Part model, mm, in its own coordinate system. A direction names the side the tool comes from. Round coordinates to 2 decimals unless told otherwise and drop trailing zeros. Order: outer loops, then holes, each group sorted by start corner. A loop starts at its lowest first (then second) coordinate and runs counter-clockwise, first axis right, second up. Notation, with made-up numbers: M 85.25,74 L 103.25,74 A15 ccw 103.25,100 Z; hole C -31,55.5 d2. An arc over 180 degrees is marked long. Write each question's results on one line, items separated by ' | '. Start each with the question number.
1. Band-saw the part on B-B, the plane z = -64. List the corners of the cut face in (x, y), then the cut area to 3 significant figures.
2. Probe L1, parallel to X at y = 5.75, z = -88; L2, parallel to X at y = 3.25, z = -13; L3, parallel to Z at x = 39, y = 8.25. List the from-to ranges inside material, lowest first. Write a range as [from, to].
3. Which spindle directions (+Z, -Z, +X, -X, +Y, -Y) get a long thin tool onto all of the face, cutting with end or side? Do faces 1 (the face through (6, 7, -49)), 2 (the face through (82, 7, -6)), 3 (the face through (70, 5, -88)), 4 (the face through (30, 5, -12)), 5 (the face through (18, 7, -94)). Say none if no direction does.
4. Two-plate mould, pull along X, no slides. Class faces 6 (the face through (100, 2, -49)), 7 (the face through (15, 2, 0)), 8 (the face through (50, 5, -20)): +X half, -X half, draft (parallel to the pull), parting line (faces both ways), or undercut.
5. Band-saw the part on C-C, the plane x = 11.5. List the corners of the cut face in (y, z).
6. Band-saw the part on D-D, the plane y = 3. List the corners of the cut face in (x, z).
7. Drop flat-ended pins along their axis: pin 1 Ø1.5 at (x, y) = (49, 6.5) entering from +Z; pin 2 Ø4 at (x, y) = (88, 8.5) entering from -Z; pin 3 Ø4 at (y, z) = (8.5, -66) entering from -X. Give the stop position or say it passes through.
8. Band-saw the part on A-A, the plane z = -13. List the corners of the cut face in (x, y).
```python
from build123d import *

# Parameters (mm, degrees)
SKETCH1_W           = 100
SKETCH1_H           = 100
BOSS_EXTRUDE1_DEPTH = 5
SKETCH2_W           = 88
SKETCH2_H           = 88
BOSS_EXTRUDE2_DEPTH = 5
SKETCH3_W           = 40
SKETCH3_H           = 20
CUT_EXTRUDE1_DEPTH  = 10


with BuildPart() as part:
    # Sketch1 → Boss-Extrude1 (new body)
    with BuildSketch(Plane(origin=(0, 0, 0), x_dir=(1, 0, 0), z_dir=(0, 1, 0))):
        with Locations((50, 50)):
            Rectangle(SKETCH1_W, SKETCH1_H)
    extrude(amount=BOSS_EXTRUDE1_DEPTH)

    # Sketch2 → Boss-Extrude2 (add)
    with BuildSketch(Plane(origin=(0, 5, 0), x_dir=(1, 0, 0), z_dir=(0, 1, 0))):
        with Locations((50, 50)):
            Rectangle(SKETCH2_W, SKETCH2_H)
    extrude(amount=BOSS_EXTRUDE2_DEPTH)

    # Sketch3 → Cut-Extrude1 (cut)
    with BuildSketch(Plane.XZ):
        with Locations((50, -90)):
            Rectangle(SKETCH3_W, SKETCH3_H)
        with Locations((50, -10)):
            Rectangle(SKETCH3_W, SKETCH3_H)
    extrude(amount=-CUT_EXTRUDE1_DEPTH, mode=Mode.SUBTRACT)


solid = part.part
```
Solution:
1) outline: M 0,0 L 100,0 L 100,5 L 94,5 L 94,10 L 6,10 L 6,5 L 0,5 Z | area: 940 mm^2
2) L1: [6, 30], [70, 94] | L2: [0, 30], [70, 100] | L3: [-80, -20]
3) face 1: +Z, -Z, -X, +Y | face 2: +Z, +X, -X, +Y | face 3: -Z, +Y, -Y | face 4: +Z, +Y, -Y | face 5: -Z, +X, -X, +Y
4) face 6: +X half | face 7: draft | face 8: undercut
5) outline: M 0,-100 L 5,-100 L 5,-94 L 10,-94 L 10,-6 L 5,-6 L 5,0 L 0,0 Z
6) outline: M 0,-100 L 30,-100 L 30,-80 L 70,-80 L 70,-100 L 100,-100 L 100,0 L 70,0 L 70,-20 L 30,-20 L 30,0 L 0,0 Z
7) pin 1: z = -20 | pin 2: z = -94 | pin 3: x = 6
8) outline: M 0,0 L 30,0 L 30,10 L 6,10 L 6,5 L 0,5 Z; M 70,0 L 100,0 L 100,5 L 94,5 L 94,10 L 70,10 Z
